```python
from build123d import *

# Parameters (mm, degrees)
EXTRUDE_425_DEPTH      = 5
EXTRUDE_425_DEPTH_BACK = 5
SKETCH_1_W             = 40
SKETCH_1_H             = 30
SKETCH_5_R             = 1.25
CUT_EXTRUDE_679_DEPTH  = 37.400549446
CUT_EXTRUDE_1219_DEPTH = 27.925824036
SKETCH_7_W             = 20
SKETCH_7_H             = 26
CUT_EXTRUDE_1457_DEPTH = 2.5
FILLET_1_R             = 1
FILLET_2_R             = 1
FILLET_3_R             = 5


with BuildPart() as part:
    # Эскиз1 → Extrude 425 (new, two sides: drawn at the far end of the back side and taken through both)
    with BuildSketch(Plane(origin=(0, 0, 0), x_dir=(1, 0, 0), z_dir=(0, 1, 0)).offset(-EXTRUDE_425_DEPTH_BACK)):
        Rectangle(SKETCH_1_W, SKETCH_1_H)
    extrude(amount=EXTRUDE_425_DEPTH + EXTRUDE_425_DEPTH_BACK)

    # Эскиз5 → Cut-Extrude 679 (cut, through all)
    with BuildSketch(Plane.XY.offset(15)):
        with Locations((-15, 0)):
            Circle(SKETCH_5_R)
        with Locations((15, 0)):
            Circle(SKETCH_5_R)
    extrude(amount=-CUT_EXTRUDE_679_DEPTH, mode=Mode.SUBTRACT)

    # Эскиз6 → Cut-Extrude 1219 (cut, through all)
    with BuildSketch(Plane(origin=(0, 5, 0), x_dir=(1, 0, 0), z_dir=(0, 1, 0))):
        Polygon((-8.738367733, 13), (8.738367733, 13), (0, 1.640121947), align=None)
        Polygon((10, 11.359878053), (10, -11.359878053), (1.261632267, 0), align=None)
        Polygon((-8.738367733, -13), (8.738367733, -13), (0, -1.640121947), align=None)
        Polygon((-10, 11.359878053), (-10, -11.359878053), (-1.261632267, 0), align=None)
    extrude(amount=-CUT_EXTRUDE_1219_DEPTH, mode=Mode.SUBTRACT)

    # Эскиз7 → Cut-Extrude 1457 (cut)
    with BuildSketch(Plane(origin=(0, 5, 0), x_dir=(1, 0, 0), z_dir=(0, 1, 0))):
        Rectangle(SKETCH_7_W, SKETCH_7_H)
    cut_extrude_1457 = extrude(amount=-CUT_EXTRUDE_1457_DEPTH, mode=Mode.SUBTRACT)

    # Зеркальное отражение1: Cut-Extrude 1457 across plane
    add(cut_extrude_1457.mirror(Plane.ZX), mode=Mode.SUBTRACT)

    # Скругление1
    fillet_1_edges = [part.edges().sort_by_distance(p)[0] for p in [
        (8.738367733, 0, 13),
        (-8.738367733, 0, 13),
        (-10, 0, 11.359878053),
        (-10, 0, -11.359878053),
        (-8.738367733, 0, -13),
        (8.738367733, 0, -13),
        (10, 0, -11.359878053),
        (10, 0, 11.359878053),
        (-10, -3.75, -13),
        (-10, -3.75, 13),
        (10, -3.75, 13),
        (10, -3.75, -13),
        (10, 3.75, -13),
        (-10, 3.75, -13),
        (-10, 3.75, 13),
        (10, 3.75, 13),
    ]]
    fillet(fillet_1_edges, radius=FILLET_1_R)

    # Скругление2
    fillet_2_edges = [part.edges().sort_by_distance(p)[0] for p in [
        (0, 0, 1.640121947),
        (-1.261632267, 0, 0),
        (0, 0, -1.640121947),
        (1.261632267, 0, 0),
    ]]
    fillet(fillet_2_edges, radius=FILLET_2_R)

    # Скругление3
    fillet_3_edges = [part.edges().sort_by_distance(p)[0] for p in [
        (-20, -5, 0),
        (-20, 5, 0),
        (20, -5, 0),
        (20, 5, 0),
    ]]
    fillet(fillet_3_edges, radius=FILLET_3_R - 0.0001)  # a hair under: the kernel refuses the full size


solid = part.part
```
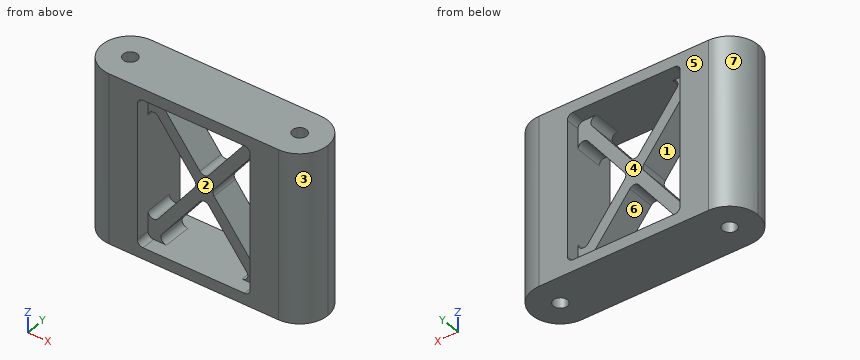
Could you check a few things on this model? Use its own coordinates, in mm. Face numbers are marked on the shaded views. A direction names the side the tool comes from. Round coordinates to 2 decimals unless told otherwise and drop trailing zeros. Write each loop counter-clockwise with the first axis right and the second up, starting at its lowest first coordinate (ties: lowest second). Pieces come first, ordered by that corner, then holes. Notation, with made-up numbers: M -39.5,66 L 0.5,66 A4 cw 0.5,70 Z; hole C 28.5,33 d4. An arc over 180 degrees is marked long. Write each question's results on one line, items separated by ' | '. Start each with the question number.
1. Imagine slicing it at B-B on x = 3. List the corners of the cut face in (y, z) for me.
2. Thinking about a two-plate mould opening in X: for the marked faces 4, 5, 6 and 7, which applies, +X half, -X half, draft (parallel to the pull), parting line (faces both ways), or undercut?
3. I'm going to push flat-ended pins straight in: pin 1 Ø2 at (x, y) = (-15, 0) entering from -Z; pin 2 Ø10 at (x, z) = (-3, -0.5) entering from +Y; pin 3 Ø16 at (x, z) = (0.5, 3.5) entering from -Y. Where does each tip first touch, or does it pass through?
4. On a 3-axis mill with a long thin cutter (end or side, diameter ignored), from which of +Z, -Z, +X, -X, +Y, -Y can I reach the whole of each face in a straight line? I mean the marked faces 1, 2 and 3. Say none if no direction works.
5. I need wall thicknesses on L1, parallel to Z at x = -4, y = 4.25; L2, parallel to Y at x = 15, z = 7.5; L3, parallel to X at y = -1.75, z = -6.25. Which ranges of each line are inside material? Lowest first, please. Write a range as from..to.
6. Imagine slicing it at A-A on z = 4. Count the separate pieces of the cut face and the enclosed holes in it, and give its area (3 significant figures).
7. Imagine slicing it at D-D on y = 4. List the corners of the cut face in (x, z) for me, and give its area (3 significant figures).
Result sheet:
1) outline: M -5,-15 L 5,-15 L 5,-13 L -5,-13 Z; M -5,13 L 5,13 L 5,15 L -5,15 Z; M -2.5,-5.54 L 2.5,-5.54 L 2.5,-2.26 L -2.5,-2.26 Z; M -2.5,2.26 L 2.5,2.26 L 2.5,5.54 L -2.5,5.54 Z
2) face 4: undercut | face 5: draft | face 6: undercut | face 7: -X half
3) pin 1: passes through | pin 2: stops at y = 2.5 | pin 3: stops at y = -2.5
4) face 1: +Y, -Y | face 2: -Y | face 3: +Z, -Z, +X, -Y
5) L1: z = -15..-13, 13..15 | L2: y = -5..-1.25, 1.25..5 | L3: x = -19.68..-10, -6.07..-3.55, 3.55..6.07, 10..19.68
6) separate pieces: 4 | enclosed holes: 2 | area: 194 mm^2
7) outline: M -18,-15 L 18,-15 L 18,15 L -18,15 Z; hole M -10,-12 A1 ccw -9,-13 L 9,-13 A1 ccw 10,-12 L 10,12 A1 ccw 9,13 L -9,13 A1 ccw -10,12 Z | area: 561 mm^2
